Verification items for the finished model (mm, model axes). Face numbers are marked on the shaded views. A direction names the side the tool comes from. Round coordinates to 2 decimals unless told otherwise and drop trailing zeros. Loops run counter-clockwise (first coordinate to the right, second up) from the corner with the lowest first, then second, coordinate; pieces in that order, holes last.
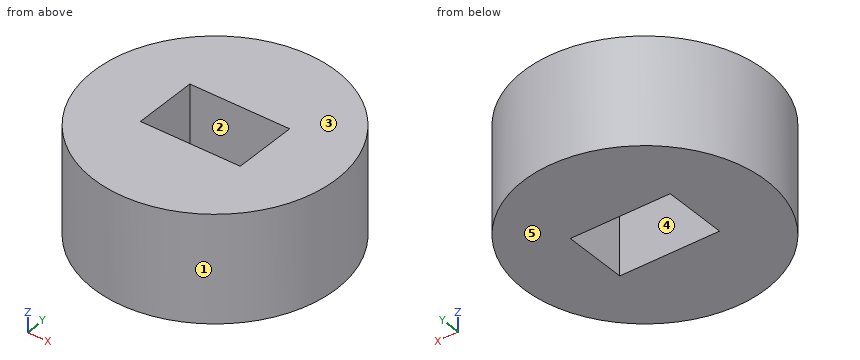
from build123d import *

# Parameters (mm, degrees)
MODEL_R                 = 3.4
MODEL_W                 = 2.8
MODEL_H                 = 1.8
SALIENTE_EXTRUIR1_DEPTH = 3


with BuildPart() as part:
    # Model → Saliente-Extruir1 (new body)
    with BuildSketch(Plane.XY):
        with Locations((12.869725503, 293.551469222)):
            Circle(MODEL_R)
        with Locations((12.869725503, 293.551469222)):
            Rectangle(MODEL_W, MODEL_H, mode=Mode.SUBTRACT)
    extrude(amount=SALIENTE_EXTRUIR1_DEPTH)


solid = part.part
1. Gauge pin test, flat ends, axial feed: P1, Ø1.5, axis at x = 11.5, z = 2.5, coming from the -Y side; P2, Ø1.5, axis at x = 15.5, z = 1.5, coming from the -Y side; P3, Ø1, axis at x = 12.5, y = 293, coming from the -Z side; P4, Ø1.5, axis at x = 15, z = 2, coming from the +Y side. Record the tip position at first contact, or that the pin passes through.
2. Section check A-A (x = 12.5). Enter the section's corners in (y, z).
3. Section check B-B (y = 293.75). Enter the section's corners in (x, z), then the cut area to 3 significant figures.
4. Release check for a two-part mould opening along Y. For the marked faces 1, 2 and 3 record: released by +Y, released by -Y, zero draft, split by the parting line, or undercut.
5. Section check D-D (y = 296). Enter the section's corners in (x, z).
6. Scan lines: L1, parallel to X at y = 293.5, z = 1.1; L2, parallel to Y at x = 13, z = 2.6; L3, parallel to Y at x = 14, z = 2.4. Record each from-to range of solid material in increasing order.
7. Section check C-C (z = 0.95). Enter the section's corners in (x, y).
8. Tool access check on the marked faces 4 and 5. Record the directions out of +Z, -Z, +X, -X, +Y, -Y that give a thin tool (end or side, any length) a straight path to the whole face; none if there is none.
Taken from the geometry:
1. P1: stops at y = 290.21
1. P2: stops at y = 290.72
1. P3: stops at z = 0
1. P4: stops at y = 296.66
2. outline: (290.17, 0) - (292.65, 0) - (292.65, 3) - (290.17, 3) - close; (294.45, 0) - (296.93, 0) - (296.93, 3) - (294.45, 3) - close
3. outline: (9.48, 0) - (11.47, 0) - (11.47, 3) - (9.48, 3) - close; (14.27, 0) - (16.26, 0) - (16.26, 3) - (14.27, 3) - close
3. area: 12.0 mm2
4. face 1: split by the parting line
4. face 2: undercut
4. face 3: zero draft
5. outline: (10.51, 0) - (15.23, 0) - (15.23, 3) - (10.51, 3) - close
6. L1: x = 9.47 to 11.47, 14.27 to 16.27
6. L2: y = 290.15 to 292.65, 294.45 to 296.95
6. L3: y = 290.34 to 292.65, 294.45 to 296.76
7. outline: circle Ø6.8 at (12.87, 293.55); hole (11.47, 292.65) - (14.27, 292.65) - (14.27, 294.45) - (11.47, 294.45) - close
8. face 4: +Z, -Z
8. face 5: -Z, +X, -X, +Y, -Y
